Model file for the job. Use its own axes, mm. Face numbers are marked on the shaded views. A direction names the side the tool comes from. Coordinates: 2 decimals unless noted, no trailing zeros. Loops run counter-clockwise (first coordinate to the right, second up) from the corner with the lowest first, then second, coordinate; pieces in that order, holes last. Notation, with made-up numbers: (-11, 54) -> (2, 54) arc R22 ccw to (2, 62) -> close; hole circle Ø11 at (-25.5, 47.5). An arc over 180 degrees is marked (long way). Use one line per item in the form item = value.
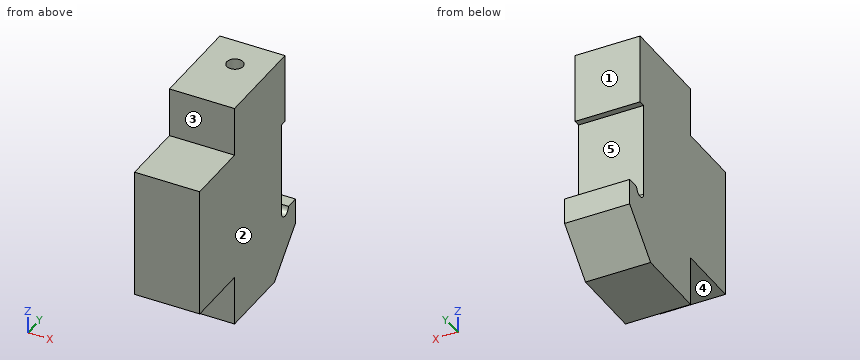
```python
from build123d import *

# Parameters (mm, degrees)
BOSS_EXTRUDE1_DEPTH       = 10
CHAMFER1_SIZE             = 6
M3X0_5_TAPPED_HOLE1_D     = 2.5
M3X0_5_TAPPED_HOLE1_DEPTH = 14.5
M3X0_5_TAPPED_HOLE1_TIP   = 0.751075774


with BuildPart() as part:
    # Sketch1 → Boss-Extrude1 (new body)
    with BuildSketch(Plane(origin=(0, 0, 0), x_dir=(0, 0, -1), z_dir=(1, 0, 0))):
        with BuildLine():
            Line((0, 1), (0, 3))
            Line((0, 3), (10, 3))
            Line((10, 3), (10, -14.46))
            Line((10, -14.46), (2.365, -14.46))
            Line((2.365, -14.46), (2.365, -24.46))
            Line((2.365, -24.46), (-17.635, -24.46))
            Line((-17.635, -24.46), (-17.635, -14.46))
            Line((-17.635, -14.46), (-25.27, -14.46))
            Line((-25.27, -14.46), (-25.27, 0))
            Line((-25.27, 0), (-14.5, 0))
            Line((-14.5, 0), (-14.5, -1))
            Line((-14.5, -1), (0, -1))
            ThreePointArc((0, -1), (1, 0), (0, 1))
        make_face()
    extrude(amount=-BOSS_EXTRUDE1_DEPTH)

    # Chamfer1
    chamfer1_edges = [part.edges().sort_by_distance(p)[0] for p in [
        (-5, 3, -10),
    ]]
    chamfer(chamfer1_edges, length=CHAMFER1_SIZE)

    # M3x0.5 Tapped Hole1
    with Locations(Plane(origin=(-5, -5, 25.27), x_dir=(1, 0, 0), z_dir=(0, 0, 1))):
        with Locations((0, 0)):
            Hole(M3X0_5_TAPPED_HOLE1_D / 2, depth=M3X0_5_TAPPED_HOLE1_DEPTH)
            with Locations((0, 0, -(M3X0_5_TAPPED_HOLE1_DEPTH + M3X0_5_TAPPED_HOLE1_TIP / 2))):  # 118° drill point
                Cone(0, M3X0_5_TAPPED_HOLE1_D / 2, M3X0_5_TAPPED_HOLE1_TIP, mode=Mode.SUBTRACT)


solid = part.part
```
Q1. Which spindle directions (+Z, -Z, +X, -X, +Y, -Y) get a long thin tool onto all of the face, cutting with end or side? Do the marked faces 1, 2, 3, 4 and 5. Say none if no direction does.
Result:
face_1 = +Z, +X, -X, +Y
face_2 = +Z, -Z, +X, +Y, -Y
face_3 = +Z, +X, -X, -Y
face_4 = -Z, +X, -X, -Y
face_5 = +X, -X, +Y
Q2. Band-saw the part on B-B, the plane x = -7.75. Write the cut outline in (y, z) (3 decimals), and give its area (3 significant figures).
Result:
outline = (-24.46, -2.365) -> (-14.46, -2.365) -> (-14.46, -10) -> (-3, -10) -> (3, -4) -> (3, 0) -> (1, 0) arc R1 cw to (-1, 0) -> (-1, 14.5) -> (0, 14.5) -> (0, 25.27) -> (-14.46, 25.27) -> (-14.46, 17.635) -> (-24.46, 17.635) -> close
area = 706 mm2
Q3. Pin check, flat tips, straight feed: pin 1 Ø1 at (x, y) = (-3.5, 2.5) entering from +Z; pin 2 Ø1.5 at (x, z) = (-1, -6.5) entering from -Y; pin 3 Ø5 at (x, y) = (-3.5, -19.5) entering from -Z (3 decimals). Stop position of each tip, or through.
Result:
pin_1 = 0
pin_2 = -14.46
pin_3 = -2.365
Q4. Band-saw the part on C-C, the plane y = 1.75. Write the cut outline in (x, z), and give its area (3 significant figures).
Result:
outline = (-10, -5.25) -> (0, -5.25) -> (0, 0) -> (-10, 0) -> close
area = 52.5 mm2
Q5. Band-saw the part on D-D, the plane z = -3. Write the cut outline in (x, y).
Result:
outline = (-10, -14.46) -> (0, -14.46) -> (0, 3) -> (-10, 3) -> close
Q6. Wall check: line 1 along X through (y, z) = (-5, 15.75); line 2 along Y through (x, z) = (-5, 20.75); line 3 along Z through (x, y) = (-4.5, -16.5) (3 decimals). Give the ranges that are in metal, low to high.
Result:
line_1 = -10 to -6.25, -3.75 to 0
line_2 = -14.46 to -6.25, -3.75 to 0
line_3 = -2.365 to 17.635
Q7. Band-saw the part on A-A, the plane z = 21. Write the cut outline in (x, y).
Result:
outline = (-10, -14.46) -> (0, -14.46) -> (0, 0) -> (-10, 0) -> close; hole circle Ø2.5 at (-5, -5)
